Input: part model. Units: mm. Frame: model coordinates. A direction names the side the tool comes from. Coordinates: 2 decimals unless noted, no trailing zeros. Loops run counter-clockwise (first coordinate to the right, second up) from the corner with the lowest first, then second, coordinate; pieces in that order, holes last. Notation, with made-up numbers: (68, 33) - (120, 33) arc R17 ccw to (120, 49) - close; hole circle Ø2 at (46, 50). An arc over 180 degrees is marked (long way). Answer as CSV lines item,"result". Start each with the question number.
```python
from build123d import *

# Parameters (mm, degrees)
SKETCH1_W                    = 76.2
SKETCH1_H                    = 101.6
BODY_DEPTH                   = 50.8
SKETCH2_W                    = 45.72
SKETCH2_H                    = 32.3088
CAMERA_HOLE_DEPTH            = 6.35
HOLLOW_START                 = -35.56
HOLLOW_DEPTH                 = 71.12
HOLLOW_2_OUTLINE_W           = 3.81
HOLLOW_2_OUTLINE_H           = 37.3888
HOLLOW_2_DEPTH               = 10.16
HOLLOW_START_2               = 25.4
HOLLOW_3_OUTLINE_W           = 3.81
HOLLOW_3_OUTLINE_H           = 37.3888
HOLLOW_3_DEPTH               = 10.16
SINGLE_BUTTON_LEG_HOLE_REACH = 121.812
ALL_BUTTON_HOLES_COUNT       = 4
SKETCH5_W                    = 50.8
SKETCH5_H                    = 101.6
LET_FOLKS_SEE_IN_DEPTH       = 2.54
F_4_40_TAPPED_HOLE1_D        = 2.2606
F_4_40_TAPPED_HOLE1_DEPTH    = 7.62
F_4_40_TAPPED_HOLE1_TIP      = 0.679152758


# Read off the part's stored shape, not the designer's step: hollow
with BuildPart() as part:
    # Sketch1 → body (new body)
    with BuildSketch(Plane.XY):
        Rectangle(SKETCH1_W, SKETCH1_H)
    extrude(amount=BODY_DEPTH)

    # Sketch2 → camera hole (cut)
    with BuildSketch(Plane(origin=(0, 50.8, 0), x_dir=(1, 0, 0), z_dir=(0, 1, 0))):
        with Locations((0, -22.264701422)):
            Rectangle(SKETCH2_W, SKETCH2_H)
    extrude(amount=-CAMERA_HOLE_DEPTH, mode=Mode.SUBTRACT)

    # hollow outline → hollow (cut)
    with BuildSketch(Plane.YZ.offset(HOLLOW_START)):
        Polygon((48.26, 40.959101422), (48.26, 48.26), (-48.26, 48.26), (-48.26, 2.54), (48.26, 2.54), (48.26, 3.570301422), (44.45, 3.570301422), (44.45, 40.959101422), align=None)
    extrude(amount=HOLLOW_DEPTH, mode=Mode.SUBTRACT)

    # hollow 2 outline → hollow 2 (cut)
    with BuildSketch(Plane.YZ.offset(HOLLOW_START)):
        with Locations((46.355, 22.264701422)):
            Rectangle(HOLLOW_2_OUTLINE_W, HOLLOW_2_OUTLINE_H)
    extrude(amount=HOLLOW_2_DEPTH, mode=Mode.SUBTRACT)

    # hollow 3 outline → hollow 3 (cut)
    with BuildSketch(Plane.YZ.offset(HOLLOW_START_2)):
        with Locations((46.355, 22.264701422)):
            Rectangle(HOLLOW_3_OUTLINE_W, HOLLOW_3_OUTLINE_H)
    extrude(amount=HOLLOW_3_DEPTH, mode=Mode.SUBTRACT)

    # Sketch4 → single button leg hole (cut, up to next)
    with BuildSketch(Plane.XZ.offset(50.8), mode=Mode.PRIVATE) as single_button_leg_hole_sk1:
        with BuildLine():
            Line((8.128, 20.955), (8.128, 17.145))
            ThreePointArc((8.128, 17.145), (6.35, 15.367), (4.572, 17.145))
            Line((4.572, 17.145), (4.572, 20.955))
            ThreePointArc((4.572, 20.955), (6.35, 22.733), (8.128, 20.955))
        make_face()
    single_button_leg_hole_tool1 = extrude(single_button_leg_hole_sk1.sketch, amount=-SINGLE_BUTTON_LEG_HOLE_REACH, mode=Mode.PRIVATE) & part.part
    single_button_leg_hole = single_button_leg_hole_tool1.solids().sort_by_distance((6.35, -50.8, 19.05))[0]
    add(single_button_leg_hole, mode=Mode.SUBTRACT)

    # all button holes: single button leg hole ×4 about axis
    all_button_holes_axis = Axis((0, 0, 19.05), (0, 1, 0))
    for i in range(1, ALL_BUTTON_HOLES_COUNT):
        add(single_button_leg_hole.rotate(all_button_holes_axis, i * 360 / ALL_BUTTON_HOLES_COUNT), mode=Mode.SUBTRACT)

    # Sketch5 → let folks see in (cut)
    with BuildSketch(Plane(origin=(38.1, 0, 0), x_dir=(0, 0, -1), z_dir=(1, 0, 0))):
        with Locations((-25.4, 0)):
            Rectangle(SKETCH5_W, SKETCH5_H)
    extrude(amount=-LET_FOLKS_SEE_IN_DEPTH, mode=Mode.SUBTRACT)

    # #4-40 Tapped Hole1
    with Locations(Plane(origin=(0, 50.8, 0), x_dir=(1, 0, 0), z_dir=(0, 1, 0))):
        with Locations((-25.4, -22.86), (25.4, -22.816885961)):
            Hole(F_4_40_TAPPED_HOLE1_D / 2, depth=F_4_40_TAPPED_HOLE1_DEPTH)
            with Locations((0, 0, -(F_4_40_TAPPED_HOLE1_DEPTH + F_4_40_TAPPED_HOLE1_TIP / 2))):  # 118° drill point
                Cone(0, F_4_40_TAPPED_HOLE1_D / 2, F_4_40_TAPPED_HOLE1_TIP, mode=Mode.SUBTRACT)


solid = part.part
```
Item 1: Section query D-D, the plane y = 35. Output: boundary loops of the cut face in (x, z), and give its area (3 significant figures).
Item 2: Section query C-C, the plane z = 25.4. Output: boundary loops of the cut face in (x, y), and give its area (3 significant figures).
Item 3: Section query A-A, the plane x = 6.35. Output: boundary loops of the cut face in (y, z), and give its area (3 significant figures).
Item 4: Material intervals for probe 1 along X at (y, z) = (48.5, 22.86); probe 2 along Y at (x, z) = (24, 10); probe 3 along Z at (x, y) = (13, 21.5), sorted ascending.
Item 5: Contact query for flat-ended pins moving along their axis: P1, Ø4, axis at y = 36, z = 6, coming from the +X side; P2, Ø1.9, axis at y = 46.5, z = 36, coming from the +X side; P3, Ø7, axis at x = -9.5, y = 48, coming from the -Z side; P4, Ø3, axis at x = -10.5, z = 24.5, coming from the +Y side. Output: stop coordinate, or through.
Item 6: Set-up query: faces 1 (the cylindrical face through (6.311, -49.548, 22.733)), 2 (the flat face through (0, 1, 48.26)), 3 (the flat face through (0, 48, 6.11)), 4 (the flat face through (-25.4, 46, 13)). Return all of +Z, -Z, +X, -X, +Y, -Y with unobstructed straight access to the full face (end or side cutting, diameter ignored); none if empty.
Item 7: Section query B-B, the plane z = 33. Output: boundary loops of the cut face in (x, y).
Item 8: Draft query along Z for faces 5 (the flat face through (-2, 1, 0)), 6 (the cylindrical face through (3.683, -49.548, 25.439)), 7 (the flat face through (-38.1, -1, 25)). Return one class per face: pulls with the +Z half, pulls with the -Z half, needs draft (parallel to the pull), parting line crosses it, or undercut.
Response values:
1,outline,"(-38.1, 0) - (35.56, 0) - (35.56, 2.54) - (-35.56, 2.54) - (-35.56, 48.26) - (35.56, 48.26) - (35.56, 50.8) - (-38.1, 50.8) - close"
1,area,"490 mm²"
2,outline,"(-38.1, -50.8) - (-3.68, -50.8) - (-3.68, -48.26) - (-35.56, -48.26) - (-35.56, 48.26) - (-25.4, 48.26) - (-25.4, 44.45) - (-22.86, 44.45) - (-22.86, 50.8) - (-38.1, 50.8) - close; (3.68, -50.8) - (35.56, -50.8) - (35.56, -48.26) - (3.68, -48.26) - close; (22.86, 44.45) - (25.4, 44.45) - (25.4, 48.26) - (35.56, 48.26) - (35.56, 50.8) - (22.86, 50.8) - close"
2,area,"504 mm²"
3,outline,"(-50.8, 0) - (50.8, 0) - (50.8, 6.11) - (44.45, 6.11) - (44.45, 3.57) - (48.26, 3.57) - (48.26, 2.54) - (-48.26, 2.54) - (-48.26, 15.37) - (-50.8, 15.37) - close; (-50.8, 22.73) - (-48.26, 22.73) - (-48.26, 48.26) - (48.26, 48.26) - (48.26, 40.96) - (44.45, 40.96) - (44.45, 38.42) - (50.8, 38.42) - (50.8, 50.8) - (-50.8, 50.8) - close"
3,area,"667 mm²"
4,probe 1,"x = -38.1 to -26.53, -24.27 to -22.86, 22.86 to 24.27, 26.53 to 35.56"
4,probe 2,"y = -50.8 to -48.26, 44.45 to 50.8"
4,probe 3,"z = 0 to 2.54, 48.26 to 50.8"
5,P1,"stops at x = -35.56"
5,P2,"stops at x = 25.4"
5,P3,"stops at z = 0"
5,P4,"stops at y = -48.26"
6,face 1,"+Y, -Y"
6,face 2,"+X"
6,face 3,"+Y"
6,face 4,"none"
7,outline,"(-38.1, -50.8) - (35.56, -50.8) - (35.56, -48.26) - (-35.56, -48.26) - (-35.56, 48.26) - (-25.4, 48.26) - (-25.4, 44.45) - (-22.86, 44.45) - (-22.86, 50.8) - (-38.1, 50.8) - close; (22.86, 44.45) - (25.4, 44.45) - (25.4, 48.26) - (35.56, 48.26) - (35.56, 50.8) - (22.86, 50.8) - close"
8,face 5,"pulls with the -Z half"
8,face 6,"undercut"
8,face 7,"needs draft"
